Study the drawing (mm; zero at the part's minimum x, y, z) and answer. A direction names the side the tool comes from. Round coordinates to 2 decimals unless told otherwise and drop trailing zeros. Write each loop counter-clockwise with the first axis right and the second up, starting at its lowest first coordinate (ties: lowest second). Pieces come first, ordered by that corner, then holes. Notation, with made-up numbers: (-22, 11.25) - (30, 11.25) arc R24 ccw to (30, 26.25) - close; hole circle Ø10 at (40, 55.5). An arc over 180 degrees is marked (long way). Use one line per item in the form item = value. Start each with the question number.
1) For the marked faces 1 and 2, determine the directions among +Z, -Z, +X, -X, +Y, -Y from which every point of the face is accessible in a straight line to the end or side of a thin tool.
2) The part is cut by section A-A, the plane x = 1.25. Give the vertices of the cut face in (y, z).
3) For a pull along X with two mould halves and no side action, classify the marked faces 3, 4, 5 and 6 as released by +X, released by -X, zero draft, split by the parting line, or undercut.
4) The part is cut by section B-B, the plane z = 2.5. Give the vertices of the cut face in (x, y).
5) Consider line 1 along Z through (x, y) = (6.5, 17.5); line 2 along X through (y, z) = (17.25, 3.6); line 3 along Z through (x, y) = (4, 2). Determine where each line is inside the solid, lowest interval first. Write a range as from..to.
6) The part is cut by section C-C, the plane y = 5.5. Give the vertices of the cut face in (x, z).
7) The part is cut by section D-D, the plane y = 21. Give the vertices of the cut face in (x, z).
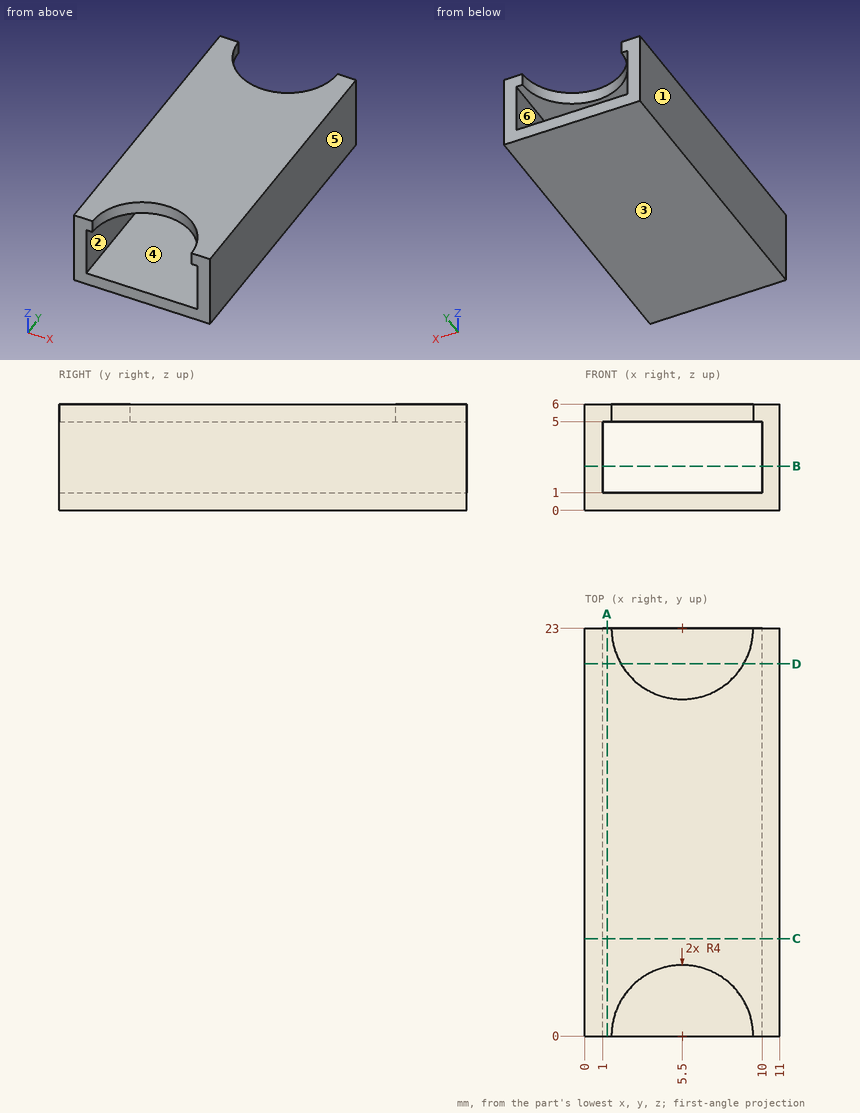
Geometry results:
q1.face_1 = +Z, -Z, -X, +Y, -Y
q1.face_2 = +Y, -Y
q2.outline = (0, 0) - (23, 0) - (23, 1) - (0, 1) - close; (0, 5) - (23, 5) - (23, 6) - (0, 6) - close
q3.face_3 = zero draft
q3.face_4 = undercut
q3.face_5 = released by +X
q3.face_6 = undercut
q4.outline = (0, 0) - (1, 0) - (1, 23) - (0, 23) - close; (10, 0) - (11, 0) - (11, 23) - (10, 23) - close
q5.line_1 = 0..1, 5..6
q5.line_2 = 0..1, 10..11
q5.line_3 = 0..1
q6.outline = (0, 0) - (11, 0) - (11, 6) - (0, 6) - close; hole (1, 1) - (10, 1) - (10, 5) - (1, 5) - close
q7.outline = (0, 0) - (11, 0) - (11, 6) - (8.96, 6) - (8.96, 5) - (10, 5) - (10, 1) - (1, 1) - (1, 5) - (2.04, 5) - (2.04, 6) - (0, 6) - close
